Design review of the part built by this model. Coordinates are the model's own, in mm. Face numbers are marked on the shaded views. A direction names the side the tool comes from. Give positions to 0.01 mm unless a question says otherwise; leave off trailing zeros. Write each loop counter-clockwise with the first axis right and the second up, starting at its lowest first coordinate (ties: lowest second). Pieces come first, ordered by that corner, then holes. Notation, with made-up numbers: M -11,18 L 39,18 A12 ccw 39,31 Z; hole C -34.5,67 d9. An arc over 180 degrees is marked long. Answer in a Markdown table with one row per item.
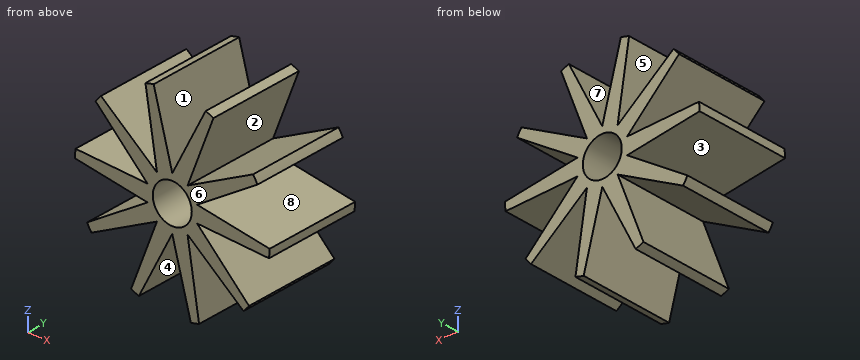
Autodesk Inventor part; units mm, degrees
ref_plane "YZ Plane" through (0, 0, 0) normal (1, 0, 0) x (0, 1, 0)
ref_plane "XZ Plane" through (0, 0, 0) normal (0, 1, 0) x (-1, 0, 0)
ref_plane "XY Plane" through (0, 0, 0) normal (0, 0, 1) x (1, 0, 0)
sketch "Sketch1" plane through (0, 0, 0) normal (0, 1, 0) x (-1, 0, 0)
  circle A0 centre (0, 0) radius 5
  line L0 (1.7129, -4.6974) -> (0.0019, -1.3369)
  line L1 (0.0019, -1.3369) -> (-0.9539, -4.9082)
  line L2 (4.1469, -2.7935) -> (0.7874, -1.0805)
  line L3 (0.7874, -1.0805) -> (2.1132, -4.5315)
  line L4 (4.9968, 0.1775) -> (1.2721, -0.4113)
  line L5 (1.2721, -0.4113) -> (4.3732, -2.4239)
  line L6 (3.9382, 3.0807) -> (1.2709, 0.4149)
  line L7 (1.2709, 0.4149) -> (4.9627, 0.6095)
  line L8 (1.3753, 4.8071) -> (0.7843, 1.0827)
  line L9 (0.7843, 1.0827) -> (3.6567, 3.4101)
  line L10 (-1.7129, 4.6974) -> (-0.0019, 1.3369)
  line L11 (-0.0019, 1.3369) -> (0.9539, 4.9082)
  line L12 (-4.1469, 2.7935) -> (-0.7874, 1.0805)
  line L13 (-0.7874, 1.0805) -> (-2.1132, 4.5315)
  line L14 (-4.9968, -0.1775) -> (-1.2721, 0.4113)
  line L15 (-1.2721, 0.4113) -> (-4.3732, 2.4239)
  line L16 (-3.9382, -3.0807) -> (-1.2709, -0.4149)
  line L17 (-1.2709, -0.4149) -> (-4.9627, -0.6095)
  line L18 (-1.3753, -4.8071) -> (-0.7843, -1.0827)
  line L19 (-0.7843, -1.0827) -> (-3.6567, -3.4101)
  dimension "d0" = 10
  dimension "d3" = 360
extrude "Extrusion1" add sketch "Sketch1" along normal blind 5 contours L4 L5 A0 L2 L3 L0 L1 L18 L19 L16 L17 L14 L15 L12 L13 L10 L11 L8 L9 L6 L7
sketch "Sketch2" plane through (0, 5, 0) normal (0, 1, 0) x (1, 0, 0)
  circle A0 centre (0, 0) radius 1
  dimension "d7" = 2
extrude "Extrusion2" cut sketch "Sketch2" against normal blind 5
properties part number "10ToothGear"
1) To check wall thickness, follow probe 1 along X at (y, z) = (1.4, 2.5); probe 2 along X at (y, z) = (4.25, -2.5); probe 3 along X at (y, z) = (2.25, 3.25). State the ranges of each line that lie inside material, in increasing order. Write a range as [from, to].
Geometry says:
| item | result |
|---|---|
| probe 1 | [-3.36, -2.53], [-1.01, -0.31], [0.59, 1.33], [3.57, 4.33] |
| probe 2 | [-4.33, -3.57], [-1.33, -0.59], [0.31, 1.01], [2.53, 3.36] |
| probe 3 | [-3.8, -3.46], [-1.13, -0.51], [0.98, 1.62] |
2) Insertion check: P1, Ø1, axis at x = -2, y = 1.5, coming from the +Z side; P2, Ø3, axis at x = 1, y = 4, coming from the +Z side; P3, Ø2, axis at y = 3.5, z = 2, coming from the +X side. Each pin has a flat end and moves straight along its axis. Give the tip position at first contact, or say it passes through.
Geometry says:
| item | result |
|---|---|
| P1 | z = 2.47 |
| P2 | z = 4.7 |
| P3 | x = 4.37 |
3) Add section A-A (z = -3.25). Write out the cut boundary in (x, y), and give its area (3 significant figures).
Geometry says:
| item | result |
|---|---|
| outline | M -1.62,0 L -0.98,0 L -0.98,5 L -1.62,5 Z; M 0.51,0 L 1.13,0 L 1.13,5 L 0.51,5 Z; M 3.46,0 L 3.8,0 L 3.8,5 L 3.46,5 Z |
| area | 8.02 mm^2 |
4) Add section B-B (x = -3.5). Write out the cut boundary in (y, z).
Geometry says:
| item | result |
|---|---|
| outline | M 0,-2.46 L 5,-2.46 L 5,-1.86 L 0,-1.86 Z; M 0,-0.06 L 5,-0.06 L 5,0.53 L 0,0.53 Z; M 0,2.64 L 5,2.64 L 5,3.28 L 0,3.28 Z |
5) For the marked faces 1, 2, 3 and 4, list the 3-axis set-ups (+Z, -Z, +X, -X, +Y, -Y) from which the entire face can be reached by the end or side of a thin tool; tool diameter is ignored.
Geometry says:
| item | result |
|---|---|
| face 1 | +Z, +Y, -Y |
| face 2 | +Y, -Y |
| face 3 | -X, +Y, -Y |
| face 4 | -Z, +Y, -Y |
6) The part is to be moulded in two halves that separate along X. For the marked faces 5, 6, 7 and 8, say which applies: released by +X, released by -X, zero draft, split by the parting line, or undercut.
Geometry says:
| item | result |
|---|---|
| face 5 | undercut |
| face 6 | zero draft |
| face 7 | undercut |
| face 8 | released by +X |
7) Add section D-D (x = -0.25). Write out the cut boundary in (y, z).
Geometry says:
| item | result |
|---|---|
| outline | M 0,-1.82 L 5,-1.82 L 5,-0.97 L 0,-0.97 Z; M 0,0.97 L 5,0.97 L 5,2.28 L 0,2.28 Z |
